Part print with two shaded views. Sizes in mm from the minimum x, y, z corner. Round coordinates to 2 decimals unless told otherwise and drop trailing zeros. Loops run counter-clockwise (first coordinate to the right, second up) from the corner with the lowest first, then second, coordinate; pieces in that order, holes last.
(1) Cut at A-A on x = 10. List the corners of the cut face in (y, z).
(2) Mould opens along X. For the marked faces 1, 2 and 3 say: +X half, -X half, draft (parallel to the pull), parting line (faces both ways), or undercut.
(3) Probe probe 1 along Y at (x, z) = (10, 2.55); probe 2 along Z at (x, y) = (5.5, 8); probe 3 along X at (y, z) = (17, 27.5). List the from-to ranges inside material, lowest first.
(4) Cut at D-D on z = 27.5. List the corners of the cut face in (x, y), then the cut area to 3 significant figures.
(5) Flat gauge pins, fed straight in: pin 1 (6 mm diameter, centred on x = 14, y = 8, fed in from -Z); pin 2 (5 mm diameter, centred on y = 17, z = 22.5, fed in from -X); pin 3 (1.5 mm diameter, centred on y = 13.5, z = 17.5, fed in from +X); pin 4 (1.5 mm diameter, centred on y = 18, z = 6.5, fed in from -X). Where does each tip first touch, or does it go through?
(6) Cut at B-B on y = 15. List the corners of the cut face in (x, z).
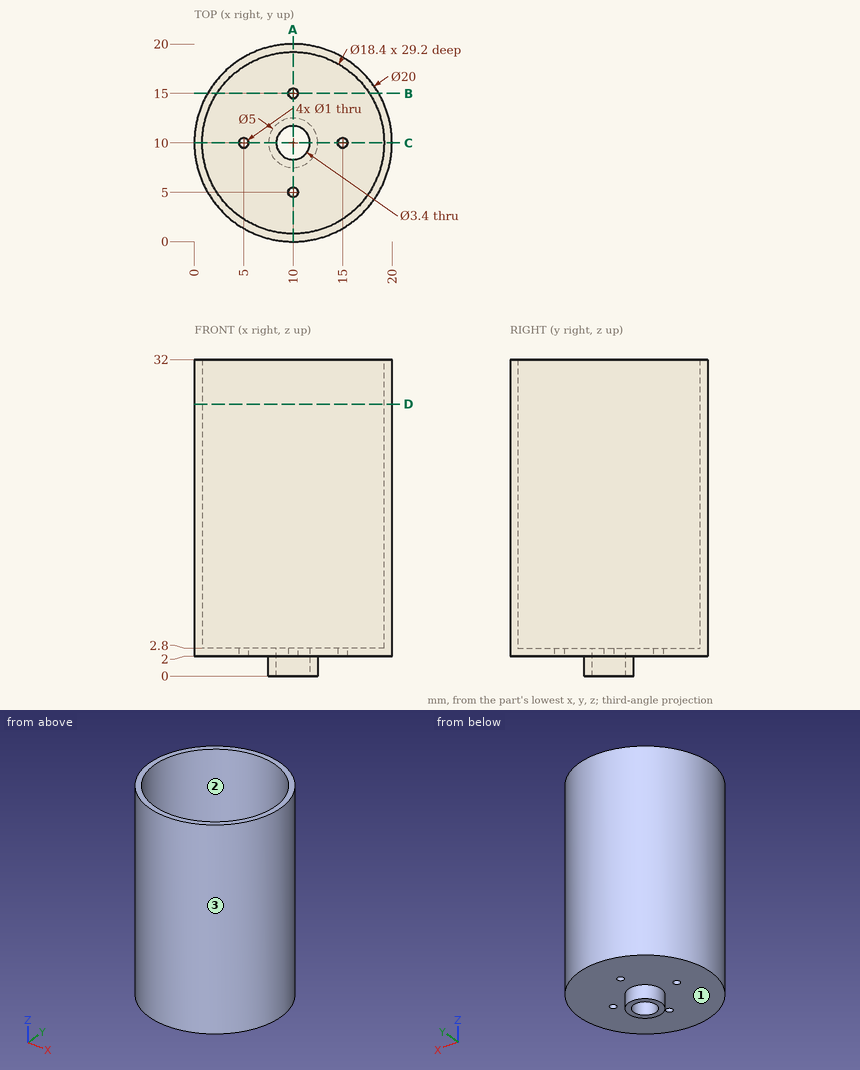
Final values:
1. outline: (0, 2) - (4.5, 2) - (4.5, 2.8) - (0.8, 2.8) - (0.8, 32) - (0, 32) - close; (5.5, 2) - (7.5, 2) - (7.5, 0) - (8.3, 0) - (8.3, 2.8) - (5.5, 2.8) - close; (11.7, 0) - (12.5, 0) - (12.5, 2) - (14.5, 2) - (14.5, 2.8) - (11.7, 2.8) - close; (15.5, 2) - (20, 2) - (20, 32) - (19.2, 32) - (19.2, 2.8) - (15.5, 2.8) - close
2. face 1: draft
2. face 2: undercut
2. face 3: parting line
3. probe 1: y = 0 to 4.5, 5.5 to 8.3, 11.7 to 14.5, 15.5 to 20
3. probe 2: z = 2 to 2.8
3. probe 3: x = 2.86 to 4.03, 15.97 to 17.14
4. outline: circle Ø20 at (10, 10); hole circle Ø18.4 at (10, 10)
4. area: 48.3 mm2
5. pin 1: stops at z = 0
5. pin 2: stops at x = 1.07
5. pin 3: stops at x = 19.61
5. pin 4: stops at x = 3.11
6. outline: (1.34, 2) - (9.5, 2) - (9.5, 2.8) - (2.28, 2.8) - (2.28, 32) - (1.34, 32) - close; (10.5, 2) - (18.66, 2) - (18.66, 32) - (17.72, 32) - (17.72, 2.8) - (10.5, 2.8) - close
